Could you check a few things on this model? Use its own coordinates, in mm. A direction names the side the tool comes from. Give positions to 0.01 mm unless a question says otherwise; leave off trailing zeros. Write each loop counter-clockwise with the first axis right and the second up, starting at its lowest first coordinate (ties: lowest second). Pieces come first, ordered by that corner, then holes. Notation, with made-up numbers: (16.5, 62) - (40.5, 62) arc R23 cw to (40.5, 71) - close; hole circle Ø3 at (76, 32). An arc over 180 degrees is marked (long way). Answer in a Markdown table with one row per item.
from build123d import *

# Parameters (mm, degrees)
REVOLUTION006_ANGLE       = -180
PAD029_DEPTH              = 0.4
BODY028_PLACEMENT_ANGLE   = 180
PAD028_DEPTH              = 2.4
FUSION007_PLACEMENT_ANGLE = 60


with BuildPart() as light006:
    # Sketch044 (on Face1 of ShapeBinder013) → Revolution006 (revolve)
    with BuildSketch(Plane.XY.offset(2.4)):
        with BuildLine():
            ThreePointArc((-2.75, 0), (0, -2.75), (2.75, 0))
            Line((-2.75, 0), (2.75, 0))
        make_face()
    revolve(axis=Axis((-2.75, 0, 2.4), (1, 0, 0)), revolution_arc=REVOLUTION006_ANGLE)


with BuildPart() as body028:
    # Sketch045 (on Face1 of ShapeBinder014) → Pad029 (new body)
    with BuildSketch(Plane(origin=(0, 0, 0), x_dir=(1, 0, 0), z_dir=(0, 0, -1))):
        with BuildLine():
            Line((3.65, 1.5), (6.65, 1.5))
            Line((6.65, 1.5), (6.65, 2))
            Line((6.65, 2), (8.65, 2))
            Line((8.65, 2), (8.65, 0.2))
            Line((8.65, 0.2), (6.65, 0.2))
            Line((6.65, 0.2), (6.65, 0.7))
            Line((6.65, 0.7), (4.45, 0.7))
            Line((4.45, 0.7), (4.45, -0.2))
            ThreePointArc((4.45, -0.2), (3.8, -0.85), (4.45, -1.5))
            Line((4.45, -1.5), (-6.65, -1.5))
            Line((-6.65, -1.5), (-6.65, -1.85))
            Line((-6.65, -1.85), (-8.65, -1.85))
            Line((-8.65, -1.85), (-8.65, -0.25))
            Line((-8.65, -0.25), (-6.65, -0.25))
            Line((-6.65, -0.25), (-6.65, -0.6))
            Line((-6.65, -0.6), (-4.95, -0.6))
            Line((-4.95, -0.6), (-4.95, 1.5))
            Line((-4.95, 1.5), (3.65, 1.5))
        make_face()
    extrude(amount=-PAD029_DEPTH)


with BuildPart() as body028_1:
    # Body028 placement: moved
    add(body028.part.moved(Location((0, 0, 1.4))).rotate(Axis((0, 0, 1.4), (1, 0, 0)), BODY028_PLACEMENT_ANGLE))


with BuildPart() as led1:
    # Sketch043 → Pad028 (new body)
    with BuildSketch(Plane.XY):
        with BuildLine():
            Line((-3.65, 1.75), (-3.65, -1.75))
            ThreePointArc((-3.65, -1.75), (0, -4), (3.65, -1.75))
            Line((3.65, 1.75), (3.65, -1.75))
            ThreePointArc((3.65, 1.75), (0, 4), (-3.65, 1.75))
        make_face()
    extrude(amount=PAD028_DEPTH)

    # Fusion007: union light006, Body028
    add(light006.part)
    add(body028_1.part)


with BuildPart() as led1_1:
    # Fusion007 placement: moved
    add(led1.part.moved(Location((0, 0, -1.5))).rotate(Axis((0, 0, -1.5), (0, 0, 1)), FUSION007_PLACEMENT_ANGLE))


solid = led1_1.part
1) Imagine slicing it at A-A (x = -2.5). List the corners of the cut face in (y, z) for me, then the cut area to 3 significant figures.
Check values:
| item | result |
|---|---|
| outline | (-8.03, -0.5) - (-5.53, -0.5) - (-5.53, -0.1) - (-8.03, -0.1) - close; (-4.27, -0.5) - (-2.77, -0.5) - (-2.77, -1.5) - (3.13, -1.5) - (3.13, 0.9) - (1.15, 0.9) arc R1.15 ccw to (-1.15, 0.9) - (-2.77, 0.9) - (-2.77, -0.1) - (-4.27, -0.1) - close |
| area | 17.8 mm2 |
2) We'd pull the mould along Y, two halves only. Please class faces 1 (the face through (-2, -5, -0.1)), 2 (the face through (3.66, 6.74, -0.3)), 3 (the face through (-3.41, -8.02, -0.3)): +Y half, -Y half, draft (parallel to the pull), parting line (faces both ways), or undercut.
Check values:
| item | result |
|---|---|
| face 1 | draft |
| face 2 | undercut |
| face 3 | -Y half |
3) If I drill on line 1 (Z direction, x = 1.75, y = 2.75); line 2 (Z direction, x = -2.75, y = -3.5); line 3 (Y direction, x = -1, z = 0.15), over which ranges is the centre line in solid material (lowest first)?
Check values:
| item | result |
|---|---|
| line 1 | z = -1.5 to 0.9 |
| line 2 | z = -0.5 to -0.1 |
| line 3 | y = -3.64 to 3.9 |
4) On a 3-axis mill with a long thin cutter (end or side, diameter ignored), from which of +Z, -Z, +X, -X, +Y, -Y can I reach the whole of each face in a straight line? I mean faces 4 (the face through (2, 6, -0.5)), 5 (the face through (-2.85, -4.07, -0.3)), 6 (the face through (0, 0, -1.5)), 7 (the face through (2, 6, -0.1)), 8 (the face through (-2, -5, -0.5)). Say none if no direction works.
Check values:
| item | result |
|---|---|
| face 4 | -Z, +X, +Y |
| face 5 | +Z, -Z, -X |
| face 6 | -Z, +X, -X, +Y, -Y |
| face 7 | +Z, +X, +Y |
| face 8 | -Z, -X, -Y |
5) Imagine slicing it at C-C (x = 0.75). List the corners of the cut face in (y, z) for me.
Check values:
| item | result |
|---|---|
| outline | (-3.96, -1.5) - (3.78, -1.5) - (3.78, -0.5) - (4.3, -0.5) - (4.3, -0.1) - (3.78, -0.1) - (3.78, 0.9) - (2.65, 0.9) arc R2.65 ccw to (-2.65, 0.9) - (-3.96, 0.9) - close |
6) Will these pins go through, and if not, where does the flat tip stop? P1, Ø2, axis at x = -1.5, z = 1.5, coming from the -Y side; P2, Ø2, axis at x = -3, y = -3.5, coming from the +Z side; P3, Ø1, axis at x = 2, z = 0.5, coming from the -Y side.
Check values:
| item | result |
|---|---|
| P1 | stops at y = -3.81 |
| P2 | stops at z = 0.9 |
| P3 | stops at y = -3.73 |
7) Imagine slicing it at D-D (z = -1). List the corners of the cut face in (x, y) for me.
Check values:
| item | result |
|---|---|
| outline | (-3.34, -2.29) - (-0.31, -4.04) arc R4.09 ccw to (3.34, 2.29) - (0.31, 4.04) arc R4.09 ccw to start |
8) Imagine slicing it at B-B (y = -0.75). List the corners of the cut face in (x, z) for me, then the cut area to 3 significant figures.
Check values:
| item | result |
|---|---|
| outline | (-3.95, -1.5) - (3.93, -1.5) - (3.93, 0.9) - (2.65, 0.9) arc R2.65 ccw to (-2.65, 0.9) - (-3.95, 0.9) - close |
| area | 29.9 mm2 |
